Design review of the part built by this model. Coordinates are the model's own, in mm. A direction names the side the tool comes from. Round coordinates to 2 decimals unless told otherwise and drop trailing zeros. Loops run counter-clockwise (first coordinate to the right, second up) from the corner with the lowest first, then second, coordinate; pieces in that order, holes last. Notation, with made-up numbers: M 38,-7.75 L 49,-7.75 A16 cw 49,-1.75 Z; hole C -21.75,84.5 d7. An arc over 180 degrees is marked long. Use a Markdown table: item, result.
from build123d import *

# Parameters (mm, degrees)
F0_W     = 42.7973791957
F0_H     = 46.9045490026
F1_DEPTH = 800
F2_DEPTH = 400
F3_DEPTH = 100
F4_DEPTH = 42.8
F5_DEPTH = 370
F6_T     = -18
F7_DEPTH = 6


with BuildPart() as f1:
    # F0 (on Top) → F1 (new body)
    with BuildSketch(Plane.XY):
        with Locations((21.3986895978, -23.4522745013)):
            Rectangle(F0_W, F0_H)
    extrude(amount=F1_DEPTH)

    # F2 (add): a face of the model
    f2_faces = [f1.faces().sort_by_distance(p)[0] for p in [
        (21.3986895978, 0, 400),
    ]]
    extrude(f2_faces, amount=-F2_DEPTH)

    # F3 (add): a face of the model
    f3_faces = [f1.faces().sort_by_distance(p)[0] for p in [
        (0, -200, 400),
    ]]
    extrude(f3_faces, amount=F3_DEPTH)

    # F4 (cut): a face of the model
    f4_faces = [f1.faces().sort_by_distance(p)[0] for p in [
        (42.7973791957, -200, 400),
    ]]
    extrude(f4_faces, amount=-F4_DEPTH, mode=Mode.SUBTRACT)

    # F5 (add): a face of the model
    f5_faces = [f1.faces().sort_by_distance(p)[0] for p in [
        (-0.0026208043, -200, 400),
    ]]
    extrude(f5_faces, amount=-F5_DEPTH)

    # F6
    f6_openings = [f1.faces().sort_by_distance(p)[0] for p in [
        (-370.002621, -200, 400),
    ]]
    offset(amount=F6_T, openings=f6_openings)

    # F7 (add): a face of the model
    f7_faces = [f1.faces().sort_by_distance(p)[0] for p in [
        (-0.0026208043, -200, 400),
    ]]
    extrude(f7_faces, amount=F7_DEPTH)


solid = f1.part
1. Machinability: for faces 4 (the face through (-192, -197, 18)), 5 (the face through (5.997, -197, 394)), which of the approach directions +Z, -Z, +X, -X, +Y, -Y give a long, thin tool a straight path to every point of the face, cutting with its end or side? Answer none if there is none.
Check values:
| item | result |
|---|---|
| face 4 | -X |
| face 5 | +Z, -Z, +X, +Y, -Y |
2. Take a section at C-C on y = -239.5. Give the boundary of the cut face in (x, z), and give its area (3 significant figures).
Check values:
| item | result |
|---|---|
| outline | M -370,0 L 6,0 L 6,800 L -370,800 L -370,782 L -18,782 L -18,18 L -370,18 Z |
| area | 31,900 mm² |
3. Take a section at B-B on x = -335.5. Give the boundary of the cut face in (y, z).
Check values:
| item | result |
|---|---|
| outline | M -400,0 L 0,0 L 0,800 L -400,800 Z; hole M -382,18 L -18,18 L -18,782 L -382,782 Z |
4. Take a section at A-A on z = 383.5. Give the boundary of the cut face in (x, y), and give its area (3 significant figures).
Check values:
| item | result |
|---|---|
| outline | M -370,-400 L 6,-400 L 6,0 L -370,0 L -370,-18 L -18,-18 L -18,-382 L -370,-382 Z |
| area | 22,300 mm² |
5. The part is to be moulded in two halves that separate along Z. For faces 1 (the face through (-185, -203, 800)), 2 (the face through (-185, -400, 394)), 3 (the face through (-192, -203, 782)), say which applies: pulls with the +Z half, pulls with the -Z half, needs draft (parallel to the pull), parting line crosses it, or undercut.
Check values:
| item | result |
|---|---|
| face 1 | pulls with the +Z half |
| face 2 | needs draft |
| face 3 | undercut |
6. Insertion check: pin 1 (8 mm diameter, centred on x = -286, z = 499.5, fed in from +Y). The pin has a flat end and moves straight along its axis. Give the tip position at first contact, or say it passes through.
Check values:
| item | result |
|---|---|
| pin 1 | stops at y = 0 |
7. Wall thickness on line 1 along Y through (x, z) = (-71.5, 586.5); line 2 along Z through (x, y) = (-207, -248); line 3 along X through (y, z) = (-153, 147): over which ranges is each line inside the solid? List them lowest first. Write a range as from..to.
Check values:
| item | result |
|---|---|
| line 1 | y = -400..-382, -18..0 |
| line 2 | z = 0..18, 782..800 |
| line 3 | x = -18..6 |
